Source: CAD feature listing. Evaluate the final solid. Frame: model axes, mm. Face numbers are marked on the shaded views. A direction names the side the tool comes from. Give positions to 0.01 mm unless a question says otherwise; leave off trailing zeros. Order: outer loops, then holes, each group sorted by start corner. A loop starts at its lowest first (then second) coordinate and runs counter-clockwise, first axis right, second up.
```python
from build123d import *

# Parameters (mm, degrees)
EXTRUDE_1_DEPTH      = 20
EXTRUDE_1_DEPTH_BACK = 10
EXTRUDE_1_2_DEPTH    = 40


with BuildPart() as part:
    # 草图1 → Extrude 1 (new, two sides: drawn at the far end of the back side and taken through both)
    with BuildSketch(Plane(origin=(0, 0, 0), x_dir=(1, 0, 0), z_dir=(0, 1, 0)).offset(-EXTRUDE_1_DEPTH_BACK)):
        with BuildLine():
            Line((0, 12.5), (100, 12.5))
            ThreePointArc((100, 12.5), (112.5, 0), (100, -12.5))
            Line((100, -12.5), (0, -12.5))
            ThreePointArc((0, -12.5), (-12.5, 0), (0, 12.5))
        make_face()
    extrude(amount=EXTRUDE_1_DEPTH + EXTRUDE_1_DEPTH_BACK)

    # 草图2 → Extrude 1 2 (add)
    with BuildSketch(Plane(origin=(0, 20, 0), x_dir=(1, 0, 0), z_dir=(0, 1, 0))):
        with BuildLine():
            Line((100, 12.5), (0, 12.5))
            ThreePointArc((0, 12.5), (-12.5, 0), (0, -12.5))
            Line((0, -12.5), (100, -12.5))
            ThreePointArc((100, -12.5), (112.5, 0), (100, 12.5))
        make_face()
        with BuildLine():
            Line((100, 7.5), (0, 7.5))
            ThreePointArc((0, 7.5), (-7.5, 0), (0, -7.5))
            Line((0, -7.5), (100, -7.5))
            ThreePointArc((100, -7.5), (107.5, 0), (100, 7.5))
        make_face(mode=Mode.SUBTRACT)
    extrude(amount=EXTRUDE_1_2_DEPTH)


solid = part.part
```
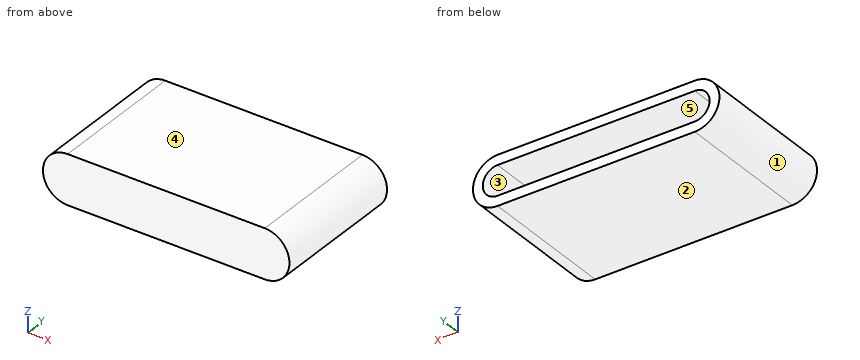
1) Section query D-D, the plane y = 9. Return the cut outline in (x, z).
Report:
outline: (0, -12.5) - (100, -12.5) arc R12.5 ccw to (100, 12.5) - (0, 12.5) arc R12.5 ccw to start
2) Reachability of the marked faces 4 and 5 from +Z, -Z, +X, -X, +Y, -Y: full face, straight path, thin tool, end or side. Return the list, or none.
Report:
face 4: +Z, +X, -X, +Y, -Y
face 5: +Y
3) Pin query (flat end, axial travel): pin 1 (5 mm diameter, centred on y = 28.5, z = 3, fed in from +X); pin 2 (1 mm diameter, centred on y = 32, z = 8, fed in from +X); pin 3 (1.5 mm diameter, centred on y = 40.5, z = -9.5, fed in from +X). Return the tip coordinate at first contact, or that it passes through.
Report:
pin 1: stops at x = 112.49
pin 2: stops at x = 110
pin 3: stops at x = 108.93
4) Draft query along X for the marked faces 1, 2 and 3. Return one class per face: +X half, -X half, draft (parallel to the pull), parting line (faces both ways), or undercut.
Report:
face 1: -X half
face 2: draft
face 3: undercut
5) Section query B-B, the plane x = 94. Return the cut outline in (y, z).
Report:
outline: (-10, -12.5) - (60, -12.5) - (60, -7.5) - (20, -7.5) - (20, 7.5) - (60, 7.5) - (60, 12.5) - (-10, 12.5) - close
6) Section query A-A, the plane y = 44.5. Return the cut outline in (x, z).
Report:
outline: (0, -12.5) - (100, -12.5) arc R12.5 ccw to (100, 12.5) - (0, 12.5) arc R12.5 ccw to start; hole (0, -7.5) - (100, -7.5) arc R7.5 ccw to (100, 7.5) - (0, 7.5) arc R7.5 ccw to start
7) Material intervals for L1, parallel to Z at x = 10.5, y = 53.5; L2, parallel to Y at x = 98, z = -6.25; L3, parallel to X at y = 29.5, z = 9, sorted ascending.
Report:
L1: z = -12.5 to -7.5, 7.5 to 12.5
L2: y = -10 to 20
L3: x = -8.67 to 108.67
8) Section query C-C, the plane z = -1.5. Return the cut outline in (x, y).
Report:
outline: (-12.41, -10) - (112.41, -10) - (112.41, 60) - (107.35, 60) - (107.35, 20) - (-7.35, 20) - (-7.35, 60) - (-12.41, 60) - close
